The model under review builds one solid part; all positions refer to its coordinate system, in mm. Face numbers are marked on the shaded views. A direction names the side the tool comes from. Round coordinates to 2 decimals unless told otherwise and drop trailing zeros. Order: outer loops, then holes, each group sorted by start corner. A loop starts at its lowest first (then second) coordinate and runs counter-clockwise, first axis right, second up.
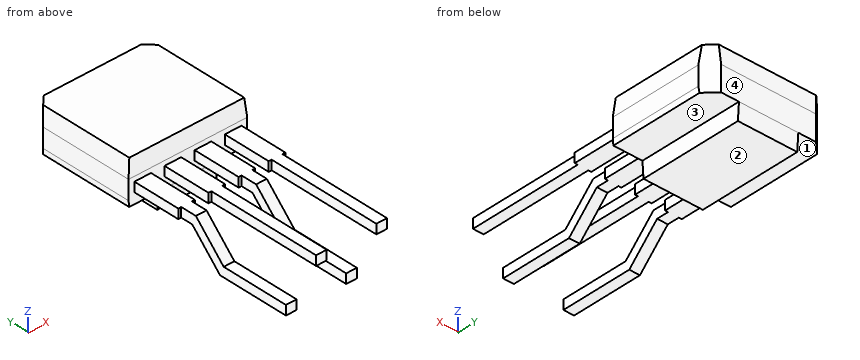
from build123d import *
from OCP.BRepFilletAPI import BRepFilletAPI_MakeChamfer

# Parameters (mm, degrees)
BOSS_EXTRUDE1_DEPTH = 4.4
CHAMFER5_SIZE       = 0.5
CHAMFER1_SIZE       = 0.25
CHAMFER1_SIZE2      = 0.026276059
CHAMFER2_SIZE       = 0.75
CHAMFER2_SIZE2      = 0.078828176
CHAMFER3_SIZE       = 0.75
CHAMFER3_SIZE2      = 0.052445109
CHAMFER4_SIZE       = 0.7
CHAMFER4_SIZE2      = 0.048948768
BOSS_EXTRUDE2_START = 0.41
BOSS_EXTRUDE2_DEPTH = 0.45
BOSS_EXTRUDE3_START = 1.68
SKETCH5_W           = 0.4
SKETCH5_H           = 6.77
BOSS_EXTRUDE3_DEPTH = 0.45
LPATTERN1_COUNT     = 2
LPATTERN1_PITCH     = 2.54
SKETCH6_W           = 0.125
SKETCH6_H           = 2
BOSS_EXTRUDE4_DEPTH = 0.4
LPATTERN2_COUNT     = 4
LPATTERN2_PITCH     = 1.27


with BuildPart() as part:
    # Sketch1 → Boss-Extrude1 (new body)
    with BuildSketch(Plane(origin=(0, 0, 0), x_dir=(1, 0, 0), z_dir=(0, 1, 0))):
        Polygon((-2.5, 0), (-2.5, 1.8), (-1.25, 1.8), (-1.25, 2.5), (1.25, 2.5), (1.25, 1.8), (2.5, 1.8), (2.5, 0), align=None)
    extrude(amount=BOSS_EXTRUDE1_DEPTH)

    # Chamfer5
    chamfer5_edges = [part.edges().sort_by_distance(p)[0] for p in [
        (-2.5, 4.4, -0.9),
        (2.5, 4.4, -0.9),
    ]]
    chamfer(chamfer5_edges, length=CHAMFER5_SIZE)

    # Chamfer1: one chamfer whose edges measure the first distance from different faces: ONE call of the kernel's chamfer builder (chamfer() names one face for all edges)
    chamfer1_edges_1 = [part.edges().sort_by_distance(p)[0] for p in [
        (2.5, 1.95, -1.8),
    ]]
    chamfer1_side_1 = [part.faces().sort_by_distance(p)[0] for p in [
        (2.5, 1.95, -0.9),
    ]]
    chamfer1_edges_2 = [part.edges().sort_by_distance(p)[0] for p in [
        (-2.5, 1.95, -1.8),
    ]]
    chamfer1_side_2 = [part.faces().sort_by_distance(p)[0] for p in [
        (-2.5, 1.95, -0.9),
    ]]
    chamfer1 = BRepFilletAPI_MakeChamfer(part.part.solid().wrapped)
    for e in chamfer1_edges_1:
        chamfer1.Add(CHAMFER1_SIZE, CHAMFER1_SIZE2, e.wrapped, chamfer1_side_1[0].wrapped)  # the first distance lies on this face
    for e in chamfer1_edges_2:
        chamfer1.Add(CHAMFER1_SIZE, CHAMFER1_SIZE2, e.wrapped, chamfer1_side_2[0].wrapped)  # the first distance lies on this face
    add(Compound.cast(chamfer1.Shape()), mode=Mode.REPLACE)

    # Chamfer2: one chamfer whose edges measure the first distance from different faces: ONE call of the kernel's chamfer builder (chamfer() names one face for all edges)
    chamfer2_edges_1 = [part.edges().sort_by_distance(p)[0] for p in [
        (2.5, 1.95, 0),
    ]]
    chamfer2_side_1 = [part.faces().sort_by_distance(p)[0] for p in [
        (2.5, 1.95, -0.775),
    ]]
    chamfer2_edges_2 = [part.edges().sort_by_distance(p)[0] for p in [
        (-2.5, 1.95, 0),
    ]]
    chamfer2_side_2 = [part.faces().sort_by_distance(p)[0] for p in [
        (-2.5, 1.95, -0.775),
    ]]
    chamfer2 = BRepFilletAPI_MakeChamfer(part.part.solid().wrapped)
    for e in chamfer2_edges_1:
        chamfer2.Add(CHAMFER2_SIZE, CHAMFER2_SIZE2, e.wrapped, chamfer2_side_1[0].wrapped)  # the first distance lies on this face
    for e in chamfer2_edges_2:
        chamfer2.Add(CHAMFER2_SIZE, CHAMFER2_SIZE2, e.wrapped, chamfer2_side_2[0].wrapped)  # the first distance lies on this face
    add(Compound.cast(chamfer2.Shape()), mode=Mode.REPLACE)

    # Chamfer3: one chamfer whose edges measure the first distance from different faces: ONE call of the kernel's chamfer builder (chamfer() names one face for all edges)
    chamfer3_edges_1 = [part.edges().sort_by_distance(p)[0] for p in [
        (0, 4.4, 0),
    ]]
    chamfer3_side_1 = [part.faces().sort_by_distance(p)[0] for p in [
        (0, 4.4, -1.144413408),
    ]]
    chamfer3_edges_2 = [part.edges().sort_by_distance(p)[0] for p in [
        (0, 0, 0),
    ]]
    chamfer3_side_2 = [part.faces().sort_by_distance(p)[0] for p in [
        (0, 0, -1.107834111),
    ]]
    chamfer3 = BRepFilletAPI_MakeChamfer(part.part.solid().wrapped)
    for e in chamfer3_edges_1:
        chamfer3.Add(CHAMFER3_SIZE, CHAMFER3_SIZE2, e.wrapped, chamfer3_side_1[0].wrapped)  # the first distance lies on this face
    for e in chamfer3_edges_2:
        chamfer3.Add(CHAMFER3_SIZE, CHAMFER3_SIZE2, e.wrapped, chamfer3_side_2[0].wrapped)  # the first distance lies on this face
    add(Compound.cast(chamfer3.Shape()), mode=Mode.REPLACE)

    # Chamfer4: one chamfer whose edges measure the first distance from different faces: ONE call of the kernel's chamfer builder (chamfer() names one face for all edges)
    chamfer4_edges_1 = [part.edges().sort_by_distance(p)[0] for p in [
        (0, 0, -2.5),
    ]]
    chamfer4_side_1 = [part.faces().sort_by_distance(p)[0] for p in [
        (0, 0, -1.493540612),
    ]]
    chamfer4_edges_2 = [part.edges().sort_by_distance(p)[0] for p in [
        (0, 4.4, -2.5),
    ]]
    chamfer4_side_2 = [part.faces().sort_by_distance(p)[0] for p in [
        (0, 4.4, -1.532352941),
    ]]
    chamfer4 = BRepFilletAPI_MakeChamfer(part.part.solid().wrapped)
    for e in chamfer4_edges_1:
        chamfer4.Add(CHAMFER4_SIZE, CHAMFER4_SIZE2, e.wrapped, chamfer4_side_1[0].wrapped)  # the first distance lies on this face
    for e in chamfer4_edges_2:
        chamfer4.Add(CHAMFER4_SIZE, CHAMFER4_SIZE2, e.wrapped, chamfer4_side_2[0].wrapped)  # the first distance lies on this face
    add(Compound.cast(chamfer4.Shape()), mode=Mode.REPLACE)

    # Sketch4 → Boss-Extrude2 (add)
    with BuildSketch(Plane(origin=(0, 0, 0), x_dir=(0, 0, -1), z_dir=(1, 0, 0)).offset(BOSS_EXTRUDE2_START)):
        Polygon((0.95, 0), (0.95, -2.665685425), (2.22, -3.935685425), (2.22, -6.77), (2.62, -6.77), (2.62, -3.77), (1.35, -2.5), (1.35, 0), align=None)
    boss_extrude2 = extrude(amount=BOSS_EXTRUDE2_DEPTH)

    # Sketch5 → Boss-Extrude3 (add)
    with BuildSketch(Plane(origin=(0, 0, 0), x_dir=(0, 0, -1), z_dir=(1, 0, 0)).offset(BOSS_EXTRUDE3_START)):
        with Locations((1.15, -3.385)):
            Rectangle(SKETCH5_W, SKETCH5_H)
    boss_extrude3 = extrude(amount=BOSS_EXTRUDE3_DEPTH)

    # LPattern1: Boss-Extrude2, Boss-Extrude3 ×2
    with Locations(*[(-i * LPATTERN1_PITCH, 0, 0) for i in range(1, LPATTERN1_COUNT)]):
        add(boss_extrude2)
        add(boss_extrude3)

    # Sketch6 → Boss-Extrude4 (add)
    with BuildSketch(Plane(origin=(0, 0, -1.35), x_dir=(-1, 0, 0), z_dir=(0, 0, -1))):
        with Locations((-2.1925, -1)):
            Rectangle(SKETCH6_W, SKETCH6_H)
        with Locations((-1.6175, -1)):
            Rectangle(SKETCH6_W, SKETCH6_H)
    boss_extrude4 = extrude(amount=-BOSS_EXTRUDE4_DEPTH)

    # LPattern2: Boss-Extrude4 ×4
    with Locations(*[(-i * LPATTERN2_PITCH, 0, 0) for i in range(1, LPATTERN2_COUNT)]):
        add(boss_extrude4)


solid = part.part
(1) To check wall thickness, follow L1, parallel to X at y = -5.75, z = -1.3; L2, parallel to X at y = -4, z = -2.4; L3, parallel to Y at x = 1.25, z = -0.9. State the ranges of each line that lie inside material, in increasing order.
(2) We need section B-B (x = 1.8). Give the boundary of the cut face in (y, z).
(3) Tool access review of the marked faces 1, 2, 3 and 4: name each direction out of +Z, -Z, +X, -X, +Y, -Y from which nothing blocks a thin tool from reaching the whole face with its end or side.
(4) We need section C-C (y = 2.25). Give the boundary of the cut face in (x, z).
(5) Clearance check with flat-ended pins moving along their axes: P1, Ø0.8, axis at x = 2, y = -3, coming from the +Z side; P2, Ø3, axis at x = 1.5, y = 2, coming from the -Z side. State where each tip first meets the part, or that it passes through.
(6) We need section D-D (x = 0.65). Give the boundary of the cut face in (y, z).
(7) We need section A-A (y = -6). Give the boundary of the cut face in (x, z).
Verdict:
1. L1: x = -0.86 to -0.41, 1.68 to 2.13
1. L2: x = -2.13 to -1.68, 0.41 to 0.86
1. L3: y = 0 to 4.4
2. outline: (-6.77, -1.35) - (0, -1.35) - (0, -1.8) - (4.4, -1.8) - (4.4, -0.75) - (4.35, 0) - (0.05, 0) - (0, -0.75) - (0, -0.95) - (-6.77, -0.95) - close
3. face 1: -Z, -X, +Y
3. face 2: -Z, +X, -X, +Y
3. face 3: -Z, +X, +Y, -Y
3. face 4: +Z, -Z, +X, -X, +Y
4. outline: (-2.5, -1.55) - (-2.47, -1.8) - (-1.25, -1.8) - (-1.25, -2.5) - (1.25, -2.5) - (1.25, -1.8) - (2.47, -1.8) - (2.5, -1.55) - (2.5, -0.75) - (2.42, 0) - (-2.42, 0) - (-2.5, -0.75) - close
5. P1: stops at z = -0.95
5. P2: stops at z = -2.5
6. outline: (-6.77, -2.62) - (-3.77, -2.62) - (-2.5, -1.35) - (0, -1.35) - (0, -1.8) - (0.05, -2.5) - (4.35, -2.5) - (4.4, -1.8) - (4.4, -0.75) - (4.35, 0) - (0.05, 0) - (0, -0.75) - (0, -0.95) - (-2.67, -0.95) - (-3.94, -2.22) - (-6.77, -2.22) - close
7. outline: (-2.13, -2.62) - (-1.68, -2.62) - (-1.68, -2.22) - (-2.13, -2.22) - close; (-0.86, -1.35) - (-0.41, -1.35) - (-0.41, -0.95) - (-0.86, -0.95) - close; (0.41, -2.62) - (0.86, -2.62) - (0.86, -2.22) - (0.41, -2.22) - close; (1.68, -1.35) - (2.13, -1.35) - (2.13, -0.95) - (1.68, -0.95) - close
